```python
from build123d import *

# Parameters (mm, degrees)
F0_R     = 55
F0_R_2   = 51
F0_R_3   = 46
F1_DEPTH = 7
F2_DEPTH = 50
F3_DEPTH = 100
F4_R     = 10


with BuildPart() as f1:
    # F0 (on Top) → F1 (new body)
    with BuildSketch(Plane.XY):
        Circle(F0_R)
        Circle(F0_R_2, mode=Mode.SUBTRACT)
        Circle(F0_R_2)
        Circle(F0_R_3, mode=Mode.SUBTRACT)
        Circle(F0_R_3)
    extrude(amount=F1_DEPTH)

    # F0 (on Top) → F2 (join)
    with BuildSketch(Plane.XY):
        Circle(F0_R_2)
        Circle(F0_R_3, mode=Mode.SUBTRACT)
    extrude(amount=-F2_DEPTH)

    # F0 (on Top) → F3 (join)
    with BuildSketch(Plane.XY):
        Circle(F0_R)
        Circle(F0_R_2, mode=Mode.SUBTRACT)
    extrude(amount=-F3_DEPTH)

    # F4
    f4_edges = [f1.edges().sort_by_distance(p)[0] for p in [
        (-55, 0, 7),
    ]]
    fillet(f4_edges, radius=F4_R)


solid = f1.part
```
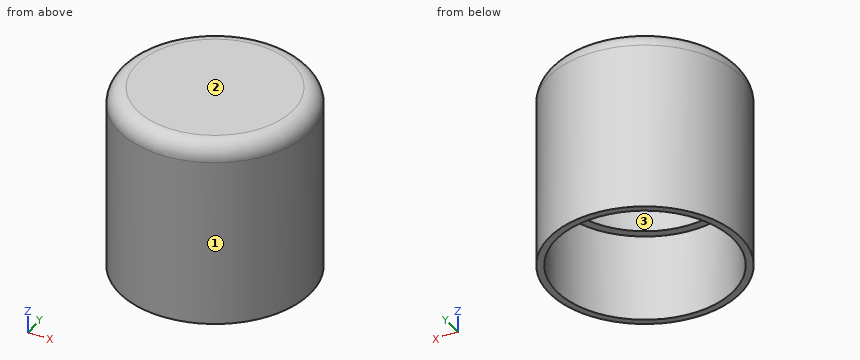
Here's how the part is built. I have some questions about the finished solid (model axes, mm). Face numbers are marked on the shaded views. Coordinates: 2 decimals unless noted, no trailing zeros. Order: outer loops, then holes, each group sorted by start corner. A loop starts at its lowest first (then second) coordinate and runs counter-clockwise, first axis right, second up.
1) We'd pull the mould along X, two halves only. Please class the marked faces 1, 2 and 3: +X half, -X half, draft (parallel to the pull), parting line (faces both ways), or undercut.
2) Imagine slicing it at A-A on y = 0. List the corners of the cut face in (x, z) for me, and give its area (3 significant figures).
3) I need wall thicknesses on line 1 (Y direction, x = 0, z = -73.5); line 2 (Z direction, x = -12, y = 2); line 3 (Y direction, x = -19, z = -68.5). Which ranges of each line are inside material? Lowest first, please.
4) Imagine slicing it at B-B on z = -36. List the corners of the cut face in (x, y) for me.
5) Imagine slicing it at D-D on z = -70.5. List the corners of the cut face in (x, y) for me, and give its area (3 significant figures).
6) Will these pins go through, and if not, where does the flat tip stop? pin 1 (6 mm diameter, centred on x = -38.5, z = -49, fed in from -Y); pin 2 (4 mm diameter, centred on x = 29, y = 39, fed in from -Z); pin 3 (1.5 mm diameter, centred on y = 7.5, z = -89, fed in from -X).
Response values:
1. face 1: parting line
1. face 2: draft
1. face 3: undercut
2. outline: (-55, -100) - (-51, -100) - (-51, -50) - (-46, -50) - (-46, 0) - (46, 0) - (46, -50) - (51, -50) - (51, -100) - (55, -100) - (55, -3) arc R10 ccw to (45, 7) - (-45, 7) arc R10 ccw to (-55, -3) - close
2. area: 2,030 mm2
3. line 1: y = -55 to -51, 51 to 55
3. line 2: z = 0 to 7
3. line 3: y = -51.61 to -47.33, 47.33 to 51.61
4. outline: circle Ø110 at (0, 0); hole circle Ø92 at (0, 0)
5. outline: circle Ø110 at (0, 0); hole circle Ø102 at (0, 0)
5. area: 1,330 mm2
6. pin 1: stops at y = -42.01
6. pin 2: stops at z = -50
6. pin 3: stops at x = -54.58
